Read the model definition and answer for the solid it produces. Units are mm, in the model's axes. A direction names the side the tool comes from. Give positions to 0.01 mm unless a question says otherwise; leave off trailing zeros. Write each loop counter-clockwise with the first axis right and the second up, starting at its lowest first coordinate (ties: lowest second). Pieces come first, ordered by that corner, then holes. Notation, with made-up numbers: (-37, 7) -> (-1, 7) arc R14 cw to (-1, 32) -> close; hole circle Ø10 at (-23, 23). An arc over 180 degrees is marked (long way). Put each result on its own line as item: value. Start each with the question number.
from build123d import *

# Parameters (mm, degrees)
BOSS_EXTRUDE1_DEPTH = 12
CUT_EXTRUDE1_DEPTH  = 80.418196907
SKETCH7_R           = 2.5
CUT_EXTRUDE2_DEPTH  = 80.418196907
SKETCH8_R           = 2.5
BOSS_EXTRUDE2_DEPTH = 15


with BuildPart() as part:
    # Sketch1 → Boss-Extrude1 (new body)
    with BuildSketch(Plane(origin=(0, 0, 0), x_dir=(0, 0, -1), z_dir=(1, 0, 0))):
        with BuildLine():
            Line((-33.5, 0), (33.5, 0))
            Line((33.5, 0), (33.5, -71))
            Line((33.5, -71), (23.5, -71))
            ThreePointArc((23.5, -71), (0, -47.5), (-23.5, -71))
            Line((-23.5, -71), (-33.5, -71))
            Line((-33.5, -71), (-33.5, 0))
        make_face()
    extrude(amount=BOSS_EXTRUDE1_DEPTH)

    # Sketch6 → Cut-Extrude1 (cut, through all)
    with BuildSketch(Plane(origin=(12, 0, 0), x_dir=(0, 0, -1), z_dir=(1, 0, 0))):
        with BuildLine():
            Line((20, 12.5), (20, -12.5))
            ThreePointArc((20, -12.5), (0, -32.5), (-20, -12.5))
            Line((-20, -12.5), (-20, 12.5))
            ThreePointArc((-20, 12.5), (0, 32.5), (20, 12.5))
        make_face()
    extrude(amount=-CUT_EXTRUDE1_DEPTH, mode=Mode.SUBTRACT)

    # Sketch7 → Cut-Extrude2 (cut, through all)
    with BuildSketch(Plane(origin=(12, 0, 0), x_dir=(0, 0, -1), z_dir=(1, 0, 0))):
        with Locations((-25.5, -35.5)):
            Circle(SKETCH7_R)
    extrude(amount=-CUT_EXTRUDE2_DEPTH, mode=Mode.SUBTRACT)

    # Sketch8 → Boss-Extrude2 (add)
    with BuildSketch(Plane(origin=(12, 0, 0), x_dir=(0, 0, -1), z_dir=(1, 0, 0))):
        with BuildLine():
            Line((-19, 1), (-34.5, 1))
            Line((-34.5, 1), (-34.5, -72))
            Line((-34.5, -72), (-22.477766793, -72))
            ThreePointArc((-22.477766793, -72), (0, -48.5), (22.477766793, -72))
            Line((22.477766793, -72), (34.5, -72))
            Line((34.5, -72), (34.5, 1))
            Line((34.5, 1), (19, 1))
            Line((19, 1), (19, -12.5))
            ThreePointArc((19, -12.5), (0, -31.5), (-19, -12.5))
            Line((-19, -12.5), (-19, 1))
        make_face()
        with Locations((-25.5, -35.5)):
            Circle(SKETCH8_R, mode=Mode.SUBTRACT)
    extrude(amount=-BOSS_EXTRUDE2_DEPTH)


solid = part.part
1) A cutting plane is placed at C-C on z = 25.5. Give the vertices of the cut face in (x, y).
2) Each of these flat-tipped pins is pushed along its axis until it touches: pin 1 Ø6 at (x, z) = (5, 17) entering from -Y; pin 2 Ø1 at (x, z) = (2, 11) entering from +Y. Where does it stop, or does it pass through?
3) A cutting plane is placed at B-B on x = 6.75. Give the vertices of the cut face in (y, z).
4) For faces 1 (the face through (5, -72, -28)), 2 (the face through (5, -6, 19)), determine the directions among +Z, -Z, +X, -X, +Y, -Y from which every point of the face is accessible in a straight line to the end or side of a thin tool.
5) A cutting plane is placed at D-D on z = 10. Give the vertices of the cut face in (x, y).
6) A cutting plane is placed at A-A on y = -35.5. Give the vertices of the cut face in (x, z).
7) For a pull along Y with two mould halves and no side action, classify faces 3 (the face through (5, -72, 29)), 4 (the face through (4.61, -33.81, 27.34)), 5 (the face through (5, -6, -19)), 6 (the face through (4.605, -31.495, -0.418)) as pulls with the +Y half, pulls with the -Y half, needs draft (parallel to the pull), parting line crosses it, or undercut.
8) Straight lines are drawn through the part: line 1 (Y direction, x = 5.25, z = 25.5); line 2 (Z direction, x = -0.25, y = -13); line 3 (Y direction, x = 10.5, z = 0.5). For each, find the intervals that lie inside material, in ascending order. Write a range as [from, to].
Results found:
1. outline: (-3, -72) -> (12, -72) -> (12, -38) -> (-3, -38) -> close; (-3, -33) -> (12, -33) -> (12, 1) -> (-3, 1) -> close
2. pin 1: stops at y = -60.69
2. pin 2: stops at y = -27.62
3. outline: (-72, -34.5) -> (1, -34.5) -> (1, -19) -> (-12.5, -19) arc R19 cw to (-12.5, 19) -> (1, 19) -> (1, 34.5) -> (-72, 34.5) -> (-72, 22.48) arc R22.5 cw (long way) to (-72, -22.48) -> close; hole circle Ø5 at (-35.5, 25.5)
4. face 1: +Z, -Z, +X, -X, -Y
4. face 2: +X, -X, +Y
5. outline: (-3, -50.84) -> (12, -50.84) -> (12, -28.66) -> (-3, -28.66) -> close
6. outline: (-3, -34.5) -> (12, -34.5) -> (12, 23) -> (-3, 23) -> close; (-3, 28) -> (12, 28) -> (12, 34.5) -> (-3, 34.5) -> close
7. face 3: pulls with the -Y half
7. face 4: undercut
7. face 5: needs draft
7. face 6: pulls with the +Y half
8. line 1: y = [-72, -38], [-33, 1]
8. line 2: z = [-34.5, -18.99], [18.99, 34.5]
8. line 3: y = [-48.51, -31.49]
